```python
from build123d import *

# Parameters (mm, degrees)
F0_R     = 19.05
F1_DEPTH = 38.1
F0_R_2   = 6.35
F2_DEPTH = 31.75
F3_DEPTH = 25.4


with BuildPart() as f1:
    # F0 (on Top) → F1 (new body)
    with BuildSketch(Plane.XY):
        with BuildLine():
            ThreePointArc((-93.689878, -12.069013), (-77.173734, -3.926966), (-70.499011, 13.234736))
            ThreePointArc((-70.499011, 13.234736), (-76.950951, 30.150144), (-93.029012, 38.472072))
            ThreePointArc((-93.029012, 38.472072), (-121.29684, 13.566834), (-93.689878, -12.069013))
        make_face()
        with Locations((-95.899011, 13.234736)):
            Circle(F0_R, mode=Mode.SUBTRACT)
    extrude(amount=F1_DEPTH)



with BuildPart() as f2:
    # F0 (on Top) → F2 (new body)
    with BuildSketch(Plane.XY):
        with BuildLine():
            ThreePointArc((43.800989, 11.574107), (40.575019, 20.031811), (32.535988, 24.192775))
            ThreePointArc((32.535988, 24.192775), (18.402075, 11.740156), (32.205555, -1.077768))
            ThreePointArc((32.205555, -1.077768), (40.463627, 2.993256), (43.800989, 11.574107))
        make_face()
        with Locations((31.100989, 11.574107)):
            Circle(F0_R_2, mode=Mode.SUBTRACT)
    extrude(amount=F2_DEPTH)


with BuildPart() as f1_1:
    add(f1.part)

    add(f2.part)  # F3 merges F2
    # F0 (on Top) → F3 (join)
    with BuildSketch(Plane.XY):
        with BuildLine():
            ThreePointArc((-93.029012, 38.472072), (-76.950951, 30.150144), (-70.499011, 13.234736))
            ThreePointArc((-70.499011, 13.234736), (-77.173734, -3.926966), (-93.689878, -12.069013))
            Line((-93.689878, -12.069013), (32.205555, -1.077768))
            ThreePointArc((32.205555, -1.077768), (18.402075, 11.740156), (32.535988, 24.192775))
            Line((32.535988, 24.192775), (-93.029012, 38.472072))
        make_face()
        with BuildLine():
            ThreePointArc((-57.799011, 5.414211), (-64.149011, 11.764211), (-57.799011, 18.114211))
            Line((-57.799011, 18.114211), (-6.999011, 18.114211))
            ThreePointArc((-6.999011, 18.114211), (-0.649011, 11.764211), (-6.999011, 5.414211))
            Line((-6.999011, 5.414211), (-57.799011, 5.414211))
        make_face(mode=Mode.SUBTRACT)
    extrude(amount=F3_DEPTH)


solid = f1_1.part
```
Input: part model. Units: mm. Frame: model coordinates. A direction names the side the tool comes from. Give positions to 0.01 mm unless a question says otherwise; leave off trailing zeros. Order: outer loops, then holes, each group sorted by start corner. A loop starts at its lowest first (then second) coordinate and runs counter-clockwise, first axis right, second up.
1. Cut plane B-B (z = 14). Return loops of the section in (x, y).
Computed:
outline: (-93.69, -12.07) - (32.21, -1.08) arc R12.7 ccw to (43.8, 11.57) arc R12.7 ccw to (32.54, 24.19) - (-93.03, 38.47) arc R25.4 ccw (long way) to start; hole circle Ø38.1 at (-95.9, 13.23); hole (-57.8, 5.41) - (-7, 5.41) arc R6.35 ccw to (-7, 18.11) - (-57.8, 18.11) arc R6.35 ccw to start; hole circle Ø12.7 at (31.1, 11.57)
2. Line query: probe 1 along X at (y, z) = (13, 30.5); probe 2 along X at (y, z) = (15, 18); probe 3 along Z at (x, y) = (17, 4). Output: solid intervals per line, ascending.
Computed:
probe 1: x = -121.3 to -114.95, -76.85 to -70.5, 18.48 to 24.91, 37.29 to 43.72
probe 2: x = -121.24 to -114.87, -76.93 to -63.26, -1.54 to 25.75, 36.45 to 43.33
probe 3: z = 0 to 25.4
3. Cut plane D-D (x = -30.5). Return loops of the section in (y, z), and give its area (3 significant figures).
Computed:
outline: (-6.55, 0) - (5.41, 0) - (5.41, 25.4) - (-6.55, 25.4) - close; (18.11, 0) - (31.36, 0) - (31.36, 25.4) - (18.11, 25.4) - close
area: 640 mm2
4. Cut plane A-A (y = 2). Return loops of the section in (x, z), and give its area (3 significant figures).
Computed:
outline: (-118.68, 0) - (-111.28, 0) - (-111.28, 38.1) - (-118.68, 38.1) - close; (-80.51, 0) - (39.45, 0) - (39.45, 31.75) - (22.76, 31.75) - (22.76, 25.4) - (-73.12, 25.4) - (-73.12, 38.1) - (-80.51, 38.1) - close
area: 3,530 mm2
5. Draft query along Y for faces 1 (the face through (-33, 18.114, 13)), 2 (the face through (-29.368, 31.232, 12.522)), 3 (the face through (-31, 19, 25.4)), 4 (the face through (-109.94, 26.11, 18.78)). Return one class per face: released by +Y, released by -Y, zero draft, split by the parting line, or undercut.
Computed:
face 1: undercut
face 2: released by +Y
face 3: zero draft
face 4: undercut
6. Set-up query: faces 5 (the face through (25, 9, 31.75)), 6 (the face through (-0.65, 11.9, 12.52)), 7 (the face through (-40, 19, 0)). Return all of +Z, -Z, +X, -X, +Y, -Y with unobstructed straight access to the full face (end or side cutting, diameter ignored); none if empty.
Computed:
face 5: +Z, +X, +Y, -Y
face 6: +Z, -Z
face 7: -Z, +X, -X, +Y, -Y
7. Cut plane C-C (x = 26.5). Return loops of the section in (y, z), and give its area (3 significant figures).
Computed:
outline: (-1.58, 0) - (7.2, 0) - (7.2, 31.75) - (-0.26, 31.75) - (-0.26, 25.4) - (-1.58, 25.4) - close; (15.95, 0) - (24.88, 0) - (24.88, 25.4) - (23.41, 25.4) - (23.41, 31.75) - (15.95, 31.75) - close
area: 544 mm2
8. Pin query (flat end, axial travel): pin 1 Ø8 at (x, z) = (-4, 23.5) entering from -Y; pin 2 Ø12.5 at (x, y) = (32, 13.5) entering from +Z; pin 3 Ø6 at (y, z) = (26, 6.5) entering from -X; pin 4 Ø1 at (x, y) = (-8.5, 16.5) entering from +Z. Return the tip coordinate at first contact, or that it passes through.
Computed:
pin 1: stops at y = -4.59
pin 2: stops at z = 31.75
pin 3: stops at x = -119.35
pin 4: passes through
